Geometry: see drawing. Coordinates: mm, zero at the bounding-box minimum. A direction names the side the tool comes from. Coordinates: 2 decimals unless noted, no trailing zeros. Order: outer loops, then holes, each group sorted by start corner. A loop starts at its lowest first (then second) coordinate and runs counter-clockwise, first axis right, second up.
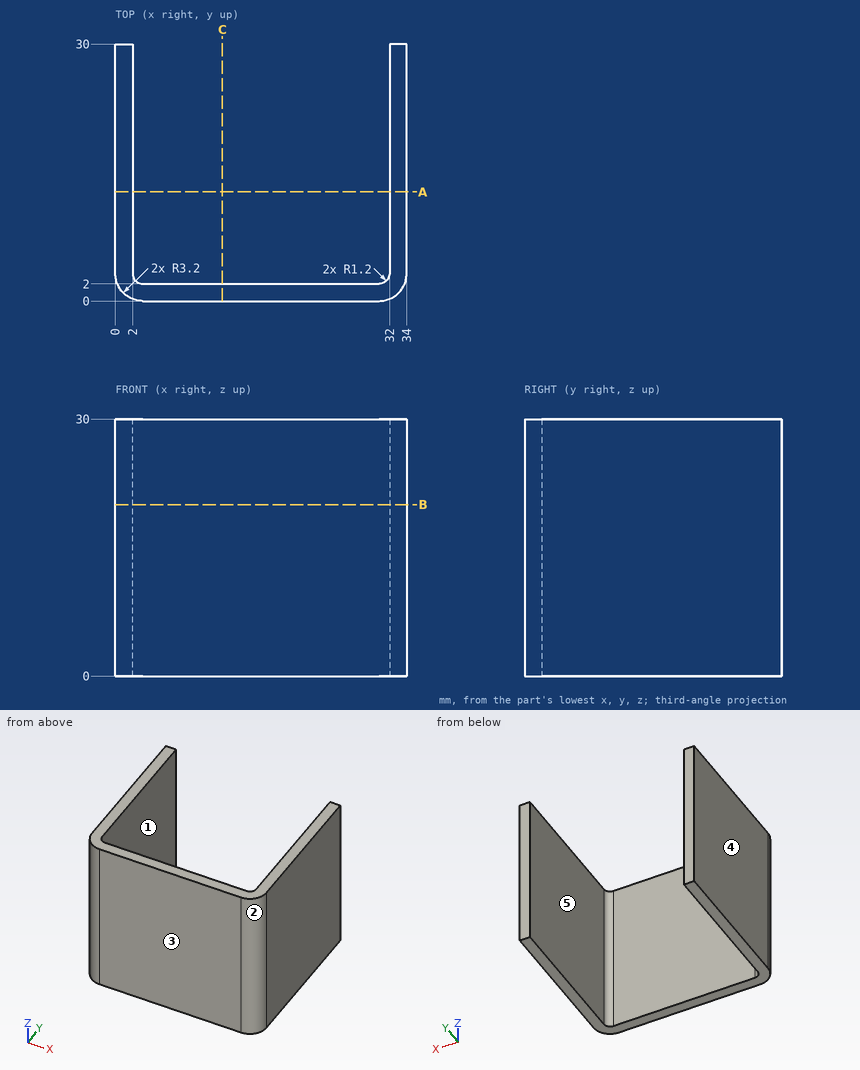
Item 1: Cut plane B-B on z = 20. Return loops of the section in (x, y), then the cut area to 3 significant figures.
Response values:
outline: (0, 3.2) arc R3.2 ccw to (3.2, 0) - (30.8, 0) arc R3.2 ccw to (34, 3.2) - (34, 30) - (32, 30) - (32, 3.2) arc R1.2 cw to (30.8, 2) - (3.2, 2) arc R1.2 cw to (2, 3.2) - (2, 30) - (0, 30) - close
area: 176 mm2
Item 2: Cut plane A-A on y = 12.75. Return loops of the section in (x, z).
Response values:
outline: (0, 0) - (2, 0) - (2, 30) - (0, 30) - close; (32, 0) - (34, 0) - (34, 30) - (32, 30) - close
Item 3: Draft query along X for the marked faces 1, 2 and 3. Return one class per face: pulls with the +X half, pulls with the -X half, needs draft (parallel to the pull), parting line crosses it, or undercut.
Response values:
face 1: undercut
face 2: pulls with the +X half
face 3: needs draft
Item 4: Cut plane C-C on x = 12.5. Return loops of the section in (y, z), then the cut area to 3 significant figures.
Response values:
outline: (0, 0) - (2, 0) - (2, 30) - (0, 30) - close
area: 60.0 mm2
Item 5: Access query for the marked faces 4 and 5. Directions: +Z, -Z, +X, -X, +Y, -Y. A direction counts if a zero-diameter tool reaches every point of the face in a straight line with its end or side. Return the directions, or none.
Response values:
face 4: +Z, -Z, -X, +Y, -Y
face 5: +Z, -Z, +Y
Item 6: Ray query, probe 1 along X at (y, z) = (25, 14.25); probe 2 along Y at (x, z) = (21, 9). Return the intervals inside material, ascending.
Response values:
probe 1: x = 0 to 2, 32 to 34
probe 2: y = 0 to 2
Item 7: Pin query (flat end, axial travel): pin 1 Ø6 at (x, z) = (13, 14) entering from +Y. Return the tip coordinate at first contact, or that it passes through.
Response values:
pin 1: stops at y = 2
